from build123d import *

# Parameters (mm, degrees)
SKETCH1_R            = 76.2
BOSS_EXTRUDE1_DEPTH  = 25.4
SKETCH2_R            = 19.05
BOSS_EXTRUDE2_DEPTH  = 63.5
CUT_EXTRUDE1_START   = -63.5
CUT_EXTRUDE1_DEPTH   = 63.5
SKETCH6_W            = 9.7550551
SKETCH6_H            = 31.75
BOSS_EXTRUDE7_DEPTH  = 31.75
CUT_EXTRUDE2_DEPTH   = 31.75
SKETCH8_R            = 9.525
CUT_EXTRUDE3_DEPTH   = 140.7
CUT_EXTRUDE4_DEPTH   = 140.7
SKETCH11_W           = 9.7550551
SKETCH11_H           = 31.75
BOSS_EXTRUDE8_DEPTH  = 31.75
CUT_EXTRUDE5_DEPTH   = 129.110325398
SKETCH13_W           = 31.75
SKETCH13_H           = 9.7550551
BOSS_EXTRUDE9_DEPTH  = 31.75
CUT_EXTRUDE6_DEPTH   = 129.110325398
SKETCH15_W           = 31.75
SKETCH15_H           = 9.7550551
BOSS_EXTRUDE10_DEPTH = 31.75
CUT_EXTRUDE7_DEPTH   = 129.110325398
SKETCH17_R           = 6.7564
CUT_EXTRUDE8_DEPTH   = 140.7


with BuildPart() as part:
    # Sketch1 → Boss-Extrude1 (new body)
    with BuildSketch(Plane.XY):
        Circle(SKETCH1_R)
    extrude(amount=BOSS_EXTRUDE1_DEPTH)

    # Sketch2 → Boss-Extrude2 (add)
    with BuildSketch(Plane(origin=(0, 0, 0), x_dir=(-1, 0, 0), z_dir=(0, 0, -1))):
        Circle(SKETCH2_R)
    extrude(amount=BOSS_EXTRUDE2_DEPTH)

    # Sketch4 → Cut-Extrude1 (cut)
    with BuildSketch(Plane(origin=(0, 0, -63.5), x_dir=(-1, 0, 0), z_dir=(0, 0, -1)).offset(CUT_EXTRUDE1_START)):
        with BuildLine():
            Line((-4.87752755, 18.415), (4.87752755, 18.415))
            ThreePointArc((4.87752755, 18.415), (0, 19.05), (-4.87752755, 18.415))
        make_face()
        with BuildLine():
            Line((-18.415, 4.87752755), (-18.415, -4.87752755))
            ThreePointArc((-18.415, -4.87752755), (-19.05, 0), (-18.415, 4.87752755))
        make_face()
        with BuildLine():
            Line((4.87752755, -18.415), (-4.87752755, -18.415))
            ThreePointArc((-4.87752755, -18.415), (0, -19.05), (4.87752755, -18.415))
        make_face()
        with BuildLine():
            Line((18.415, 4.87752755), (18.415, -4.87752755))
            ThreePointArc((18.415, -4.87752755), (19.05, 0), (18.415, 4.87752755))
        make_face()
    extrude(amount=CUT_EXTRUDE1_DEPTH, mode=Mode.SUBTRACT)

    # Sketch6 → Boss-Extrude7 (add)
    with BuildSketch(Plane(origin=(0, 0, 0), x_dir=(-1, 0, 0), z_dir=(0, 0, -1))):
        with Locations((0, 34.29)):
            Rectangle(SKETCH6_W, SKETCH6_H)
    extrude(amount=BOSS_EXTRUDE7_DEPTH)

    # Sketch7 → Cut-Extrude2 (cut)
    with BuildSketch(Plane(origin=(4.87752755, 0, 0), x_dir=(0, 0, -1), z_dir=(1, 0, 0))):
        Polygon((31.75, 18.415), (0, 50.165), (31.75, 50.165), align=None)
    extrude(amount=-CUT_EXTRUDE2_DEPTH, mode=Mode.SUBTRACT)

    # Sketch8 → Cut-Extrude3 (cut, through all)
    with BuildSketch(Plane.XY.offset(25.4)):
        Circle(SKETCH8_R)
    extrude(amount=-CUT_EXTRUDE3_DEPTH, mode=Mode.SUBTRACT)

    # Sketch9 → Cut-Extrude4 (cut, through all)
    with BuildSketch(Plane.XY.offset(25.4)):
        with BuildLine():
            Line((-2.38125, 11.90625), (-2.38125, 9.222541593))
            ThreePointArc((-2.38125, 9.222541593), (0, 9.525), (2.38125, 9.222541593))
            Line((2.38125, 9.222541593), (2.38125, 11.90625))
            Line((2.38125, 11.90625), (-2.38125, 11.90625))
        make_face()
    extrude(amount=-CUT_EXTRUDE4_DEPTH, mode=Mode.SUBTRACT)

    # Sketch11 → Boss-Extrude8 (add)
    with BuildSketch(Plane(origin=(0, 0, 0), x_dir=(-1, 0, 0), z_dir=(0, 0, -1))):
        with Locations((0, -34.29)):
            Rectangle(SKETCH11_W, SKETCH11_H)
    extrude(amount=BOSS_EXTRUDE8_DEPTH)

    # Sketch12 → Cut-Extrude5 (cut, through all)
    with BuildSketch(Plane.ZY.offset(4.87752755)):
        Polygon((-31.75, -18.415), (0, -50.165), (-31.75, -50.165), align=None)
    extrude(amount=-CUT_EXTRUDE5_DEPTH, mode=Mode.SUBTRACT)

    # Sketch13 → Boss-Extrude9 (add)
    with BuildSketch(Plane(origin=(0, 0, 0), x_dir=(-1, 0, 0), z_dir=(0, 0, -1))):
        with Locations((34.29, 0)):
            Rectangle(SKETCH13_W, SKETCH13_H)
    extrude(amount=BOSS_EXTRUDE9_DEPTH)

    # Sketch14 → Cut-Extrude6 (cut, through all)
    with BuildSketch(Plane(origin=(0, 4.87752755, 0), x_dir=(1, 0, 0), z_dir=(0, 1, 0))):
        Polygon((-18.415, 31.75), (-50.165, 0), (-50.165, 31.75), align=None)
    extrude(amount=-CUT_EXTRUDE6_DEPTH, mode=Mode.SUBTRACT)

    # Sketch15 → Boss-Extrude10 (add)
    with BuildSketch(Plane(origin=(0, 0, 0), x_dir=(-1, 0, 0), z_dir=(0, 0, -1))):
        with Locations((-34.29, 0)):
            Rectangle(SKETCH15_W, SKETCH15_H)
    extrude(amount=BOSS_EXTRUDE10_DEPTH)

    # Sketch16 → Cut-Extrude7 (cut, through all)
    with BuildSketch(Plane.XZ.offset(4.87752755)):
        Polygon((18.415, -31.75), (50.165, 0), (50.165, -31.75), align=None)
    extrude(amount=-CUT_EXTRUDE7_DEPTH, mode=Mode.SUBTRACT)

    # Sketch17 → Cut-Extrude8 (cut, through all)
    with BuildSketch(Plane.XY.offset(25.4)):
        with Locations((35.921024484, 35.921024484)):
            Circle(SKETCH17_R)
        with Locations((-35.921024484, -35.921024484)):
            Circle(SKETCH17_R)
        with Locations((-35.921024484, 35.921024484)):
            Circle(SKETCH17_R)
        with Locations((35.921024484, -35.921024484)):
            Circle(SKETCH17_R)
    extrude(amount=-CUT_EXTRUDE8_DEPTH, mode=Mode.SUBTRACT)


solid = part.part
Source: CAD feature listing. Evaluate the final solid. Frame: model axes, mm. A direction names the side the tool comes from. Round coordinates to 2 decimals unless told otherwise and drop trailing zeros. Loops run counter-clockwise (first coordinate to the right, second up) from the corner with the lowest first, then second, coordinate; pieces in that order, holes last. Notation, with made-up numbers: (39, 24) -> (94, 24) arc R6 cw to (94, 28) -> close; hole circle Ø1 at (31, -29.5). An arc over 180 degrees is marked (long way). Answer as a JSON object with one key per item and string values. Group by question number.
Q1. Mould query, pull axis X, two halves, no side actions, for faces 4 (the flat face through (-34.068, 0.068, -16.097)), 5 (the cylindrical face through (-36.8, 42.62, 12.88)), 6 (the flat face through (0, -18.415, -47)). Classes: pulls with the +X half, pulls with the -X half, needs draft (parallel to the pull), parting line crosses it, or undercut.
Q2. Section query B-B (y = 0). Output: boundary loops of the cut face in (x, z) (3 decimals), plus the area to 3 significant figures.
Q3. Section query C-C (z = -52). Output: boundary loops of the cut face in (x, y) (3 decimals), plus the area to 3 significant figures.
Q4. Section query D-D (z = 12.5). Output: boundary loops of the cut face in (x, y) (3 decimals), plus the area to 3 significant figures.
Q5. Contact query for flat-ended pins moving along their axis: P1, Ø0.8, axis at y = 11, z = -16, coming from the +X side; P2, Ø4, axis at x = 9, y = 41, coming from the -Z side; P3, Ø9.5, axis at x = -35, z = -10, coming from the +Y side. Output: stop coordinate, or through.
Q6. Access query for faces 1 (the flat face through (-4.878, 31, -12)), 2 (the flat face through (0, 18.415, -47)), 3 (the cylindrical face through (-13.37, -13.57, -31.31)). Directions: +Z, -Z, +X, -X, +Y, -Y. A direction counts if a zero-diameter tool reaches every point of the face in a straight line with its end or side. Return the directions, or none.
Q7. Section query A-A (x = 0). Output: boundary loops of the cut face in (y, z) (3 decimals).
Q8. Ray query, line 1 (Z direction, x = -69, y = -2.5); line 2 (X direction, y = 18.5, z = -24). Return the intervals inside material, ascending. Write a range as from..to.
Completed:
{
 "1": {"face 4": "pulls with the -X half", "face 5": "undercut", "face 6": "needs draft"},
 "2": {"outline": "(-76.2, 0) -> (-50.165, 0) -> (-18.415, -31.75) -> (-18.415, -63.5) -> (-9.525, -63.5) -> (-9.525, 25.4) -> (-76.2, 25.4) -> close; (9.525, -63.5) -> (18.415, -63.5) -> (18.415, -31.75) -> (50.165, 0) -> (76.2, 0) -> (76.2, 25.4) -> (9.525, 25.4) -> close", "area": "5,520 mm²"},
 "3": {"outline": "(-18.415, -4.878) arc R19.05 ccw to (-4.878, -18.415) -> (4.878, -18.415) arc R19.05 ccw to (18.415, -4.878) -> (18.415, 4.878) arc R19.05 ccw to (4.878, 18.415) -> (-4.878, 18.415) arc R19.05 ccw to (-18.415, 4.878) -> close; hole (-2.381, 9.223) arc R9.525 ccw (long way) to (2.381, 9.223) -> (2.381, 11.906) -> (-2.381, 11.906) -> close", "area": "827 mm²"},
 "4": {"outline": "circle Ø152.4 at (0, 0); hole circle Ø13.513 at (-35.921, -35.921); hole circle Ø13.513 at (-35.921, 35.921); hole (-2.381, 9.223) arc R9.525 ccw (long way) to (2.381, 9.223) -> (2.381, 11.906) -> (-2.381, 11.906) -> close; hole circle Ø13.513 at (35.921, -35.921); hole circle Ø13.513 at (35.921, 35.921)", "area": "17,400 mm²"},
 "5": {"P1": "x = 15.83", "P2": "z = 0", "P3": "y = 4.88"},
 "6": {"face 1": "-Z, -X, +Y", "face 2": "-Z, +X, -X, +Y", "face 3": "-Z, -X, -Y"},
 "7": {"outline": "(-76.2, 0) -> (-50.165, 0) -> (-18.415, -31.75) -> (-18.415, -63.5) -> (-9.525, -63.5) -> (-9.525, 25.4) -> (-76.2, 25.4) -> close; (11.906, -63.5) -> (18.415, -63.5) -> (18.415, -31.75) -> (50.165, 0) -> (76.2, 0) -> (76.2, 25.4) -> (11.906, 25.4) -> close"},
 "8": {"line 1": "0..25.4", "line 2": "-4.88..4.88"}
}
